from build123d import *

# Parameters (mm, degrees)
SKETCH_1_R             = 175
EXTRUDE_1_DEPTH        = 3
CUT_EXTRUDE_1_DEPTH    = 3
FILLET_1_R             = 5
FILLET_2_R             = 5
FILLET_3_R             = 5
SKETCH_5_R             = 1.5
CUT_EXTRUDE_4_DEPTH    = 3
SKETCH_7_W             = 30
SKETCH_7_H             = 108
CUT_EXTRUDE_6_DEPTH    = 3
SKETCH_8_R             = 1.5
CUT_EXTRUDE_7_DEPTH    = 3
SKETCH_9_R             = 1.5
CUT_EXTRUDE_8_DEPTH    = 10
SKETCH_10_R            = 1.6
CUT_EXTRUDE_9_DEPTH    = 3
SKETCH_11_W            = 15
SKETCH_11_H            = 30
CUT_EXTRUDE_10_DEPTH   = 10
SKETCH_12_R            = 1.5
CUT_EXTRUDE_11_DEPTH   = 4
SKETCH_13_R            = 1.5
CUT_EXTRUDE_12_DEPTH   = 4
PATTERN_LINEAR_1_COUNT = 2
PATTERN_LINEAR_1_PITCH = 73
SKETCH_14_R            = 1.5
CUT_EXTRUDE_14_DEPTH   = 4
SKETCH_17_R            = 1.5
CUT_EXTRUDE_15_DEPTH   = 4
SKETCH_18_R            = 1.5
CUT_EXTRUDE_16_DEPTH   = 4


with BuildPart() as part:
    # ｽｹｯﾁ1 → ﾎﾞｽ - 押し出し1 (new body)
    with BuildSketch(Plane.XY):
        Circle(SKETCH_1_R)
    extrude(amount=EXTRUDE_1_DEPTH)

    # ｽｹｯﾁ2 → ｶｯﾄ - 押し出し1 (cut)
    with BuildSketch(Plane.XY.offset(3)):
        with BuildLine():
            Line((-60, 115), (0, 115))
            Line((0, 115), (0, 175))
            ThreePointArc((0, 175), (-30.465194158, 172.327803749), (-60, 164.392822228))
            Line((-60, 164.392822228), (-60, 115))
        make_face()
        with BuildLine():
            Line((0, 175), (0, 115))
            Line((0, 115), (60, 115))
            Line((60, 115), (60, 164.392822228))
            ThreePointArc((60, 164.392822228), (30.465194158, 172.327803749), (0, 175))
        make_face()
        with BuildLine():
            Line((0, -175), (0, -115))
            Line((0, -115), (-60, -115))
            Line((-60, -115), (-60, -164.392822228))
            ThreePointArc((-60, -164.392822228), (-30.465194158, -172.327803749), (0, -175))
        make_face()
        with BuildLine():
            Line((60, -115), (0, -115))
            Line((0, -115), (0, -175))
            ThreePointArc((0, -175), (30.465194158, -172.327803749), (60, -164.392822228))
            Line((60, -164.392822228), (60, -115))
        make_face()
    extrude(amount=-CUT_EXTRUDE_1_DEPTH, mode=Mode.SUBTRACT)

    # ﾌｨﾚｯﾄ1
    fillet_1_edges = [part.edges().sort_by_distance(p)[0] for p in [
        (-60, 164.392822228, 1.5),
    ]]
    fillet(fillet_1_edges, radius=FILLET_1_R)

    # ﾌｨﾚｯﾄ2
    fillet_2_edges = [part.edges().sort_by_distance(p)[0] for p in [
        (-60, 115, 1.5),
        (60, 164.392822228, 1.5),
        (60, 115, 1.5),
    ]]
    fillet(fillet_2_edges, radius=FILLET_2_R)

    # ﾌｨﾚｯﾄ3
    fillet_3_edges = [part.edges().sort_by_distance(p)[0] for p in [
        (-60, -115, 1.5),
        (60, -115, 1.5),
        (60, -164.392822228, 1.5),
        (-60, -164.392822228, 1.5),
    ]]
    fillet(fillet_3_edges, radius=FILLET_3_R)

    # ｽｹｯﾁ5 → ｶｯﾄ - 押し出し4 (cut)
    with BuildSketch(Plane.XY.offset(3)):
        with Locations((-100, -115)):
            Circle(SKETCH_5_R)
        with Locations((100, -115)):
            Circle(SKETCH_5_R)
        with Locations((100, 115)):
            Circle(SKETCH_5_R)
        with Locations((-100, 115)):
            Circle(SKETCH_5_R)
    extrude(amount=-CUT_EXTRUDE_4_DEPTH, mode=Mode.SUBTRACT)

    # ｽｹｯﾁ7 → ｶｯﾄ - 押し出し6 (cut)
    with BuildSketch(Plane.XY.offset(3)):
        with Locations((-85, 0)):
            Rectangle(SKETCH_7_W, SKETCH_7_H)
    extrude(amount=-CUT_EXTRUDE_6_DEPTH, mode=Mode.SUBTRACT)

    # ｽｹｯﾁ8 → ｶｯﾄ - 押し出し7 (cut)
    with BuildSketch(Plane.XY.offset(3)):
        with Locations((-115, -67)):
            Circle(SKETCH_8_R)
        with Locations((-116.822468618, 0)):
            Circle(SKETCH_8_R)
        with Locations((-115, 67)):
            Circle(SKETCH_8_R)
    extrude(amount=-CUT_EXTRUDE_7_DEPTH, mode=Mode.SUBTRACT)

    # ｽｹｯﾁ9 → ｶｯﾄ - 押し出し8 (cut)
    with BuildSketch(Plane.XY.offset(3)):
        with Locations((-65, 37)):
            Circle(SKETCH_9_R)
        with Locations((20, 41)):
            Circle(SKETCH_9_R)
        with Locations((-65, -38)):
            Circle(SKETCH_9_R)
        with Locations((20, -40)):
            Circle(SKETCH_9_R)
    extrude(amount=-CUT_EXTRUDE_8_DEPTH, mode=Mode.SUBTRACT)

    # ｽｹｯﾁ10 → ｶｯﾄ - 押し出し9 (cut)
    with BuildSketch(Plane.XY.offset(3)):
        with Locations((111.643659725, -125.921059639)):
            Circle(SKETCH_10_R)
        with Locations((122.679794489, -115.037952538)):
            Circle(SKETCH_10_R)
        with Locations((168, 7.75)):
            Circle(SKETCH_10_R)
        with Locations((168, -7.75)):
            Circle(SKETCH_10_R)
        with Locations((111.56768007, 125.844011632)):
            Circle(SKETCH_10_R)
        with Locations((122.679794489, 115.037952538)):
            Circle(SKETCH_10_R)
    extrude(amount=-CUT_EXTRUDE_9_DEPTH, mode=Mode.SUBTRACT)

    # ｽｹｯﾁ11 → ｶｯﾄ - 押し出し10 (cut)
    with BuildSketch(Plane.XY.offset(3)):
        with Locations((81.317279836, 81.317279836)):
            Rectangle(SKETCH_11_W, SKETCH_11_H)
        with Locations((81.317279836, -81.317279836)):
            Rectangle(SKETCH_11_W, SKETCH_11_H)
    extrude(amount=-CUT_EXTRUDE_10_DEPTH, mode=Mode.SUBTRACT)

    # ｽｹｯﾁ12 → ｶｯﾄ - 押し出し11 (cut, through all)
    with BuildSketch(Plane.XY.offset(3)):
        with Locations((139.4, 10.5)):
            Circle(SKETCH_12_R)
        with Locations((139.4, -10.5)):
            Circle(SKETCH_12_R)
    extrude(amount=-CUT_EXTRUDE_11_DEPTH, mode=Mode.SUBTRACT)

    # ｽｹｯﾁ13 → ｶｯﾄ - 押し出し12 (cut, through all)
    with BuildSketch(Plane.XY.offset(3)):
        with Locations((50, 10)):
            Circle(SKETCH_13_R)
        with Locations((50, 64)):
            Circle(SKETCH_13_R)
        with Locations((-40, 64)):
            Circle(SKETCH_13_R)
        with Locations((-40, 10)):
            Circle(SKETCH_13_R)
        with Locations((77, 36.5)):
            Circle(SKETCH_13_R)
    cut_extrude_12 = extrude(amount=-CUT_EXTRUDE_12_DEPTH, mode=Mode.SUBTRACT)

    # 直線ﾊﾟﾀｰﾝ1: ｶｯﾄ - 押し出し12 ×2
    with Locations(*[(0, -i * PATTERN_LINEAR_1_PITCH, 0) for i in range(1, PATTERN_LINEAR_1_COUNT)]):
        add(cut_extrude_12, mode=Mode.SUBTRACT)

    # ｽｹｯﾁ14 → ｶｯﾄ - 押し出し14 (cut, through all)
    with BuildSketch(Plane.XY.offset(3)):
        with Locations((108.817279836, 89.5)):
            Circle(SKETCH_14_R)
        with Locations((108.817279836, 60)):
            Circle(SKETCH_14_R)
    extrude(amount=-CUT_EXTRUDE_14_DEPTH, mode=Mode.SUBTRACT)

    # ｽｹｯﾁ17 → ｶｯﾄ - 押し出し15 (cut, through all)
    with BuildSketch(Plane.XY.offset(3)):
        with Locations((108.817279836, -60)):
            Circle(SKETCH_17_R)
        with Locations((108.817279836, -89.5)):
            Circle(SKETCH_17_R)
    extrude(amount=-CUT_EXTRUDE_15_DEPTH, mode=Mode.SUBTRACT)

    # ｽｹｯﾁ18 → ｶｯﾄ - 押し出し16 (cut, through all)
    with BuildSketch(Plane.XY.offset(3)):
        with Locations((-135, 31.75)):
            Circle(SKETCH_18_R)
        with Locations((-135, -31.75)):
            Circle(SKETCH_18_R)
    extrude(amount=-CUT_EXTRUDE_16_DEPTH, mode=Mode.SUBTRACT)


solid = part.part
The model under review builds one solid part; all positions refer to its coordinate system, in mm. Round coordinates to 2 decimals unless told otherwise and drop trailing zeros. Return JSON: item names as keys, results as strings.
(1) For pin 1 (0.9 mm diameter, centred on y = -146.5, z = 1, fed in from +X); pin 2 (1.9 mm diameter, centred on x = 122.68, y = 115.04, fed in from +Z); pin 3 (1.5 mm diameter, centred on x = 82, z = 1.5, fed in from +Y); pin 4 (1.5 mm diameter, centred on x = 78.5, z = 1.5, fed in from -Y), all flat-tipped, find the tip position at first contact; note any pin that passes through.
Solved:
{"pin 1": "x = 96.41", "pin 2": "through", "pin 3": "y = 154.99", "pin 4": "y = -156.78"}
(2) For line 1 (X direction, y = 67, z = 1.8); line 2 (Y direction, x = 87, z = 1.5); line 3 (X direction, y = 8, z = 1.5), list the stretches that pass through material, from the lowest coordinate up.
Solved:
{"line 1": "-161.67 to -116.5, -113.5 to 73.82, 88.82 to 161.67", "line 2": "-151.84 to -96.32, -66.32 to 66.32, 96.32 to 151.84", "line 3": "-174.82 to -100, -70 to 166.42, 169.58 to 174.82"}
(3) Add section A-A on z = 2.2. State how many separate pieces and enclosed holes the cut face has, plus the area to 3 significant figures.
Solved:
{"separate pieces": "1", "enclosed holes": "38", "area": "78,200 mm2"}
